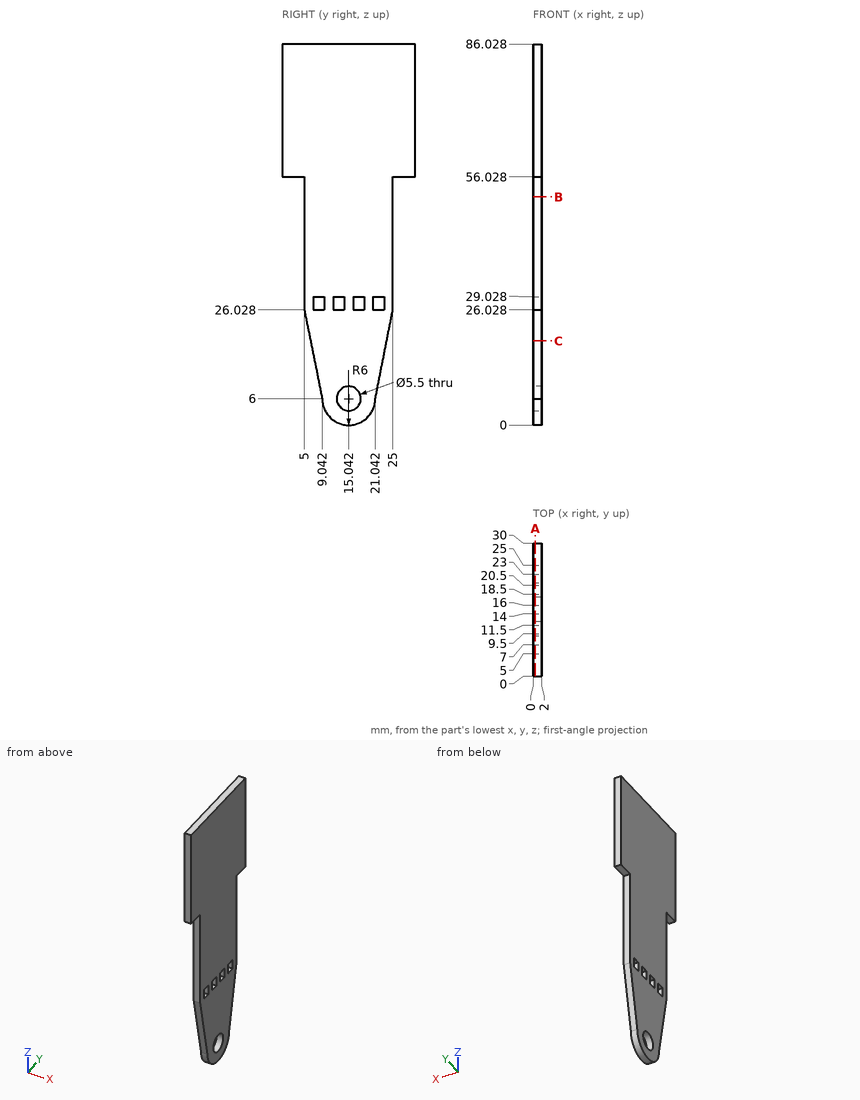
The drawing under review shows one solid part. Ordinate dimensions are in mm from its lowest x, y, z. Coordinates: 2 decimals unless noted, no trailing zeros. Loops run counter-clockwise (first coordinate to the right, second up) from the corner with the lowest first, then second, coordinate; pieces in that order, holes last.
Item 1: Wall thickness on L1, parallel to Y at x = 1.1, z = 6; L2, parallel to Z at x = 1.05, y = 16.25; L3, parallel to Z at x = 0.7, y = 17.25: over which ranges is each line inside the solid? List them lowest first.
Completed:
L1: y = 9.04 to 12.29, 17.79 to 21.04
L2: z = 0.12 to 3.53, 8.47 to 26.03, 29.03 to 86.03
L3: z = 0.42 to 4.36, 7.64 to 26.03, 29.03 to 86.03
Item 2: Add section C-C (z = 19). Write out the cut boundary in (x, y), and give its area (3 significant figures).
Completed:
outline: (0, 6.42) - (2, 6.42) - (2, 23.61) - (0, 23.61) - close
area: 34.4 mm2
Item 3: Add section B-B (z = 51.5). Write out the cut boundary in (x, y).
Completed:
outline: (0, 5) - (2, 5) - (2, 25) - (0, 25) - close
Item 4: Clearance check with flat-ended pins moving along their axes: pin 1 (1 mm diameter, centred on x = 1.5, y = 3.5, fed in from -Z); pin 2 (0.6 mm diameter, centred on x = 1, z = 27.5, fed in from +Y); pin 3 (0.6 mm diameter, centred on x = 1.5, z = 40.5, fed in from -Y). State where each tip first meets the part, or that it passes through.
Completed:
pin 1: stops at z = 56.03
pin 2: stops at y = 25
pin 3: stops at y = 5
Item 5: Add section A-A (x = 0.55). Write out the cut boundary in (y, z), and give its area (3 significant figures).
Completed:
outline: (0, 56.03) - (5, 56.03) - (5, 26.03) - (9.04, 6) arc R6 ccw to (21.04, 6) - (25, 26.03) - (25, 56.03) - (30, 56.03) - (30, 86.03) - (0, 86.03) - close; hole (7, 26.03) - (9.5, 26.03) - (9.5, 29.03) - (7, 29.03) - close; hole (11.5, 26.03) - (14, 26.03) - (14, 29.03) - (11.5, 29.03) - close; hole circle Ø5.5 at (15.04, 6); hole (16, 26.03) - (18.5, 26.03) - (18.5, 29.03) - (16, 29.03) - close; hole (20.5, 26.03) - (23, 26.03) - (23, 29.03) - (20.5, 29.03) - close
area: 1,820 mm2
